```python
from build123d import *

# Parameters (mm, degrees)
SKETCH1_W           = 100
SKETCH1_H           = 75
BOSS_EXTRUDE1_DEPTH = 65
SKETCH2_W           = 35
SKETCH2_H           = 75
CUT_EXTRUDE1_DEPTH  = 30
CUT_EXTRUDE2_DEPTH  = 40


with BuildPart() as part:
    # Sketch1 → Boss-Extrude1 (new body)
    with BuildSketch(Plane(origin=(0, 0, 0), x_dir=(1, 0, 0), z_dir=(0, 1, 0))):
        with Locations((50, 37.5)):
            Rectangle(SKETCH1_W, SKETCH1_H)
    extrude(amount=BOSS_EXTRUDE1_DEPTH)

    # Sketch2 → Cut-Extrude1 (cut)
    with BuildSketch(Plane(origin=(0, 65, 0), x_dir=(1, 0, 0), z_dir=(0, 1, 0))):
        with Locations((17.5, 37.5)):
            Rectangle(SKETCH2_W, SKETCH2_H)
    extrude(amount=-CUT_EXTRUDE1_DEPTH, mode=Mode.SUBTRACT)

    # Sketch3 → Cut-Extrude2 (cut)
    with BuildSketch(Plane(origin=(100, 0, 0), x_dir=(0, 0, -1), z_dir=(1, 0, 0))):
        with BuildLine():
            Line((25, 0), (38.28446714, 21.587259102))
            ThreePointArc((38.28446714, 21.587259102), (32.225125249, 42.861461385), (53.947292517, 47.03935034))
            Line((53.947292517, 47.03935034), (65, 65))
            Line((65, 65), (0, 65))
            Line((0, 65), (0, 0))
            Line((0, 0), (25, 0))
        make_face()
    extrude(amount=-CUT_EXTRUDE2_DEPTH, mode=Mode.SUBTRACT)


solid = part.part
```
The listing builds one solid part. Answer for the finished solid, in the listing's coordinates (mm). A direction names the side the tool comes from. Coordinates: 2 decimals unless noted, no trailing zeros. Write each loop counter-clockwise with the first axis right and the second up, starting at its lowest first coordinate (ties: lowest second). Pieces come first, ordered by that corner, then holes. Notation, with made-up numbers: (46.5, 61) - (65.5, 61) arc R19 cw to (65.5, 71) - close; hole circle Ø7 at (-26.75, 56). An arc over 180 degrees is marked (long way). One line per item, written item: value.
1) A tool of negligible diameter and unlimited length cuts with its end or side. For faces 1 (the flat face through (49, 0, -46)), 2 (the flat face through (17, 35, -38)), 3 (the flat face through (80.3, 55.9, -59.4)), from which of +Z, -Z, +X, -X, +Y, -Y can it reach the whole face along a straight path? Write none if from no direction.
Geometry check:
face 1: +Z, -Z, +X, -X, -Y
face 2: +Z, -Z, -X, +Y
face 3: +X, +Y
2) Consider line 1 along Y through (x, z) = (19.5, -64.5); line 2 along X through (y, z) = (22, -23.5); line 3 along X through (y, z) = (50.5, -34). Determine where each line is inside the solid, lowest interval first. Write a range as from..to.
Geometry check:
line 1: y = 0..35
line 2: x = 0..60
line 3: x = 35..60
3) Find section D-D (z = -45). Give the vertices of the cut face in (x, y).
Geometry check:
outline: (0, 0) - (100, 0) - (100, 50) - (60, 50) - (60, 65) - (35, 65) - (35, 35) - (0, 35) - close
4) Each of these flat-tipped pins is pushed along its axis until it touches: pin 1 Ø5 at (y, z) = (10, -24) entering from +X; pin 2 Ø8 at (x, z) = (82, -49.5) entering from +Y; pin 3 Ø24 at (y, z) = (51.5, -20.5) entering from -X; pin 4 Ø12 at (x, y) = (61.5, 27.5) entering from +Z. Where does it stop, or does it pass through?
Geometry check:
pin 1: stops at x = 60
pin 2: stops at y = 49.99
pin 3: stops at x = 35
pin 4: stops at z = 0
5) Find section A-A (z = -33). Give the vertices of the cut face in (x, y).
Geometry check:
outline: (0, 0) - (100, 0) - (100, 13) - (60, 13) - (60, 26) - (100, 26) - (100, 44) - (60, 44) - (60, 65) - (35, 65) - (35, 35) - (0, 35) - close
6) Find section B-B (x = 89). Give the vertices of the cut face in (y, z), and give its area (3 significant figures).
Geometry check:
outline: (0, -75) - (65, -75) - (65, -65) - (47.04, -53.95) arc R15 ccw (long way) to (21.59, -38.28) - (0, -25) - close
area: 2,340 mm2
7) Find section C-C (y = 28). Give the vertices of the cut face in (x, z), and give its area (3 significant figures).
Geometry check:
outline: (0, -75) - (100, -75) - (100, -31.73) - (60, -31.73) - (60, 0) - (0, 0) - close
area: 6,230 mm2
8) For a pull along Y with two mould halves and no side action, classify faces 4 (the flat face through (0, 17, -37)), 5 (the cylindrical face through (80.28, 42.563, -32.046)), 6 (the flat face through (53, 65, -38)), 7 (the flat face through (80.28, 10.64, -31.55)) as pulls with the +Y half, pulls with the -Y half, needs draft (parallel to the pull), parting line crosses it, or undercut.
Geometry check:
face 4: needs draft
face 5: undercut
face 6: pulls with the +Y half
face 7: undercut
